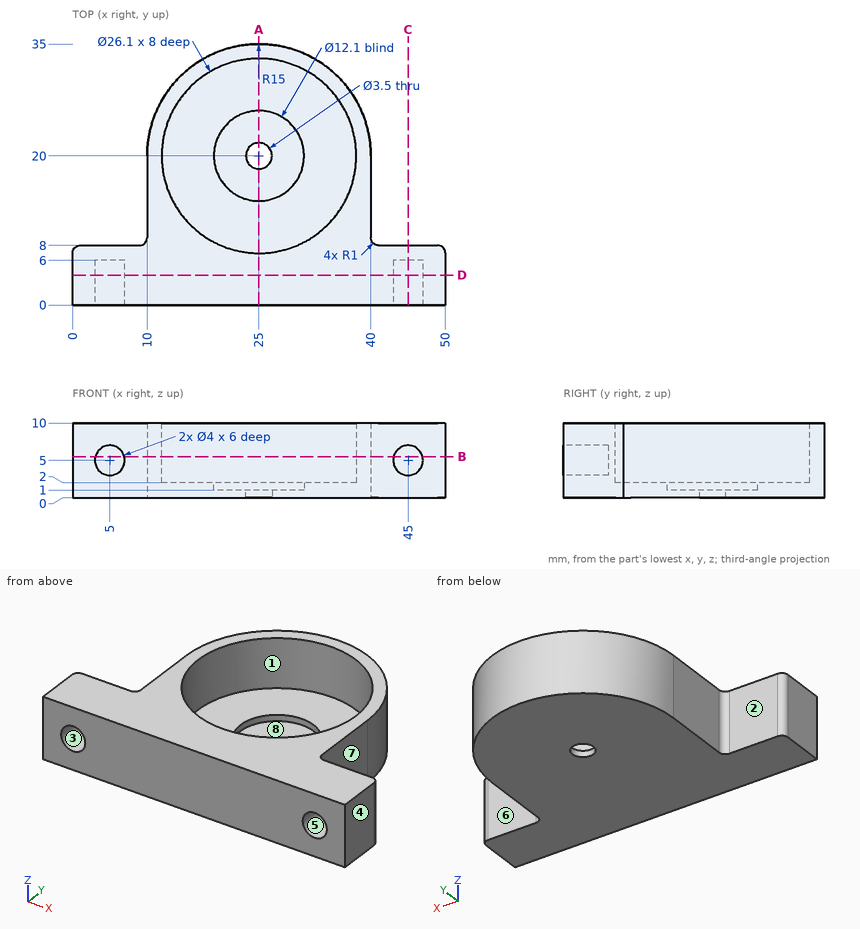
The drawing under review shows one solid part. Ordinate dimensions are in mm from its lowest x, y, z. A direction names the side the tool comes from. Round coordinates to 2 decimals unless told otherwise and drop trailing zeros. Loops run counter-clockwise (first coordinate to the right, second up) from the corner with the lowest first, then second, coordinate; pieces in that order, holes last. Notation, with made-up numbers: (0.25, 28.5) - (11.25, 28.5) arc R30 cw to (11.25, 62.5) - close; hole circle Ø7 at (63.25, -30). An arc over 180 degrees is marked (long way). Use one line per item in the form item = value.
Item 1: Tool access review of the marked faces 1, 2, 3 and 4: name each direction out of +Z, -Z, +X, -X, +Y, -Y from which nothing blocks a thin tool from reaching the whole face with its end or side.
Answers:
face_1 = +Z
face_2 = +Z, -Z, -X, +Y
face_3 = -Y
face_4 = +Z, -Z, +X, +Y, -Y
Item 2: For line 1 (Z direction, x = 5, y = 3.1); line 2 (Y direction, x = 25, z = 0.45); line 3 (Y direction, x = 25, z = 8.25), list the stretches that pass through material, from the lowest coordinate up.
Answers:
line_1 = 0 to 3, 7 to 10
line_2 = 0 to 18.25, 21.75 to 35
line_3 = 0 to 6.95, 33.05 to 35
Item 3: Consider section B-B on z = 5.5. Write out the cut boundary in (x, y).
Answers:
outline = (0, 0) - (3.06, 0) - (3.06, 6) - (6.94, 6) - (6.94, 0) - (43.06, 0) - (43.06, 6) - (46.94, 6) - (46.94, 0) - (50, 0) - (50, 7) arc R1 ccw to (49, 8) - (41, 8) arc R1 cw to (40, 9) - (40, 20) arc R15 ccw to (10, 20) - (10, 9) arc R1 cw to (9, 8) - (1, 8) arc R1 ccw to (0, 7) - close; hole circle Ø26.1 at (25, 20)
Item 4: Consider section C-C on x = 45. Write out the cut boundary in (y, z), then the cut area to 3 significant figures.
Answers:
outline = (0, 0) - (8, 0) - (8, 10) - (0, 10) - (0, 7) - (6, 7) - (6, 3) - (0, 3) - close
area = 56.0 mm^2
Item 5: Mouldability with a two-part tool opening along X and no side actions: class the marked faces 5, 6, 7 and 8 as +X half, -X half, draft (parallel to the pull), parting line (faces both ways), or undercut.
Answers:
face_5 = undercut
face_6 = draft
face_7 = +X half
face_8 = undercut
Item 6: Consider section A-A on x = 25. Write out the cut boundary in (y, z), then the cut area to 3 significant figures.
Answers:
outline = (0, 0) - (18.25, 0) - (18.25, 1) - (13.95, 1) - (13.95, 2) - (6.95, 2) - (6.95, 10) - (0, 10) - close; (21.75, 0) - (35, 0) - (35, 10) - (33.05, 10) - (33.05, 2) - (26.05, 2) - (26.05, 1) - (21.75, 1) - close
area = 126 mm^2
Item 7: Consider section D-D on y = 4. Write out the cut boundary in (x, z), then the cut area to 3 significant figures.
Answers:
outline = (0, 0) - (50, 0) - (50, 10) - (0, 10) - close; hole circle Ø4 at (5, 5); hole circle Ø4 at (45, 5)
area = 475 mm^2
Item 8: Clearance check with flat-ended pins moving along their axes: P1, Ø5, axis at x = 45, z = 5, coming from the +Y side; P2, Ø3, axis at y = 16.5, z = 5, coming from the -X side; P3, Ø6, axis at x = 23, y = 18.5, coming from the +Z side; P4, Ø2, axis at x = 25, y = 20, coming from the -Z side. State where each tip first meets the part, or that it passes through.
Answers:
P1 = 8
P2 = 10
P3 = 1
P4 = through
